Answer from the drawing. Dimensions are ordinates in mm from the lowest x, y and z of the part. A direction names the side the tool comes from. Give positions to 0.01 mm unless a question says otherwise; leave off trailing zeros. Order: outer loops, then holes, each group sorted by start corner. A loop starts at its lowest first (then second) coordinate and runs counter-clockwise, first axis right, second up. Notation, with made-up numbers: (-13, 66) - (7, 66) arc R25 cw to (7, 87) - close; hole circle Ø6 at (48.5, -39). An arc over 180 degrees is marked (long way). One line per item, written item: value. Start each with the question number.
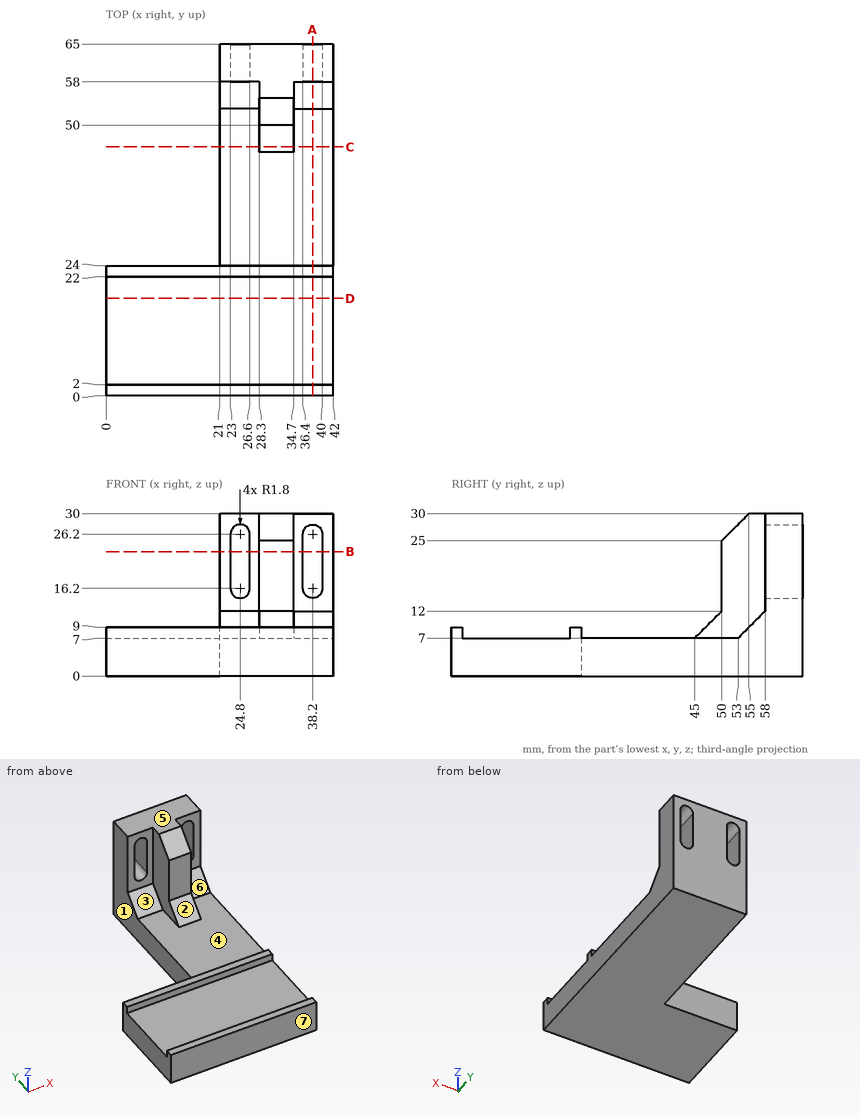
1) Find the intervals of material crossed by probe 1 along Y at (x, z) = (5.5, 7.75); probe 2 along Z at (x, y) = (27, 5); probe 3 along Y at (x, z) = (10, 3.25), in increasing order. Write a range as from..to.
2) For the marked faces 1, 2, 3 and 4, determine the directions among +Z, -Z, +X, -X, +Y, -Y from which every point of the face is accessible in a straight line to the end or side of a thin tool.
3) The mould has two halves that part along Y. Classify the marked faces 5, 6 and 7: +Y half, -Y half, draft (parallel to the pull), parting line (faces both ways), or undercut.
4) Section A-A on x = 38.2 is taken. Write down the section's boundary in (y, z).
5) Section C-C on y = 46 is taken. Write down the section's boundary in (x, z), plus the area to 3 significant figures.
6) Section D-D on y = 18 is taken. Write down the section's boundary in (x, z).
7) Each of these flat-tipped pins is pushed along its axis until it touches: pin 1 (4 mm diameter, centred on x = 17.5, y = 23, fed in from -Z); pin 2 (4.5 mm diameter, centred on x = 15.5, z = 4.5, fed in from +Y); pin 3 (7 mm diameter, centred on x = 32.5, z = 21.5, fed in from -Y); pin 4 (4 mm diameter, centred on y = 50.5, z = 16, fed in from +X). Where does it stop, or does it pass through?
8) Section B-B on z = 23 is taken. Write down the section's boundary in (x, y).
Solved:
1. probe 1: y = 0..2, 22..24
1. probe 2: z = 0..7
1. probe 3: y = 0..24
2. face 1: +Z, -Z, -X, +Y
2. face 2: +Z, +X, -X
2. face 3: +Z, -X
2. face 4: +Z
3. face 5: draft
3. face 6: undercut
3. face 7: -Y half
4. outline: (0, 0) - (65, 0) - (65, 14.4) - (58, 14.4) - (58, 12) - (53, 7) - (24, 7) - (24, 9) - (22, 9) - (22, 7) - (2, 7) - (2, 9) - (0, 9) - close; (58, 28) - (65, 28) - (65, 30) - (58, 30) - close
5. outline: (21, 0) - (42, 0) - (42, 7) - (34.7, 7) - (34.7, 8) - (28.3, 8) - (28.3, 7) - (21, 7) - close
5. area: 153 mm2
6. outline: (0, 0) - (42, 0) - (42, 7) - (0, 7) - close
7. pin 1: stops at z = 0
7. pin 2: stops at y = 24
7. pin 3: stops at y = 50
7. pin 4: stops at x = 34.7
8. outline: (21, 58) - (23, 58) - (23, 65) - (21, 65) - close; (26.6, 58) - (28.3, 58) - (28.3, 50) - (34.7, 50) - (34.7, 58) - (36.4, 58) - (36.4, 65) - (26.6, 65) - close; (40, 58) - (42, 58) - (42, 65) - (40, 65) - close
